Could you check a few things on this drawing? It's one solid part, dimensions in mm from its lowest x, y, z. A direction names the side the tool comes from. Coordinates: 2 decimals unless noted, no trailing zeros. Order: outer loops, then holes, each group sorted by start corner. A loop starts at its lowest first (then second) coordinate and runs counter-clockwise, first axis right, second up. Notation, with made-up numbers: (56.25, 76.25) - (111.25, 76.25) arc R20 cw to (111.25, 112.25) - close; hole circle Ø4 at (8, 64). An arc over 180 degrees is marked (long way). Return JSON: item names as keys, results as strings. Group by question number.
1) Imagine slicing it at A-A (z = 6). Write out the boundary of the cut face in (x, y).
2) Which directions (+Z, -Z, +X, -X, +Y, -Y) give clear straight access to the entire face, cutting with the end or side of a thin tool? Please do the marked faces 1 and 2.
3) Imagine slicing it at B-B (y = 6.25). Write out the boundary of the cut face in (x, z), and give its area (3 significant figures).
4) For pin 1 Ø6 at (y, z) = (2.5, 21.5) entering from +X; pin 2 Ø10 at (x, z) = (8, 23.5) entering from -Y; pin 3 Ø4 at (y, z) = (5.5, 60) entering from +X, each with a flat end and sliding along its axis, tell me the tip position at first contact or that it passes through.
5) If we mould it in two halves opening along Y, with no side actions, what happens to the marked faces 3, 4 and 5? For each: pulls with the +Y half, pulls with the -Y half, needs draft (parallel to the pull), parting line crosses it, or undercut.
6) If I drill on line 1 along Y through (x, z) = (43, 43); line 2 along Y through (x, z) = (16, 51.5); line 3 along X through (y, z) = (4.75, 20.5), over which ranges is the centre line in solid material (lowest first)?
7) Imagine slicing it at D-D (x = 27.94). Write out the boundary of the cut face in (y, z).
8) Imagine slicing it at C-C (x = 38). Write out the boundary of the cut face in (y, z).
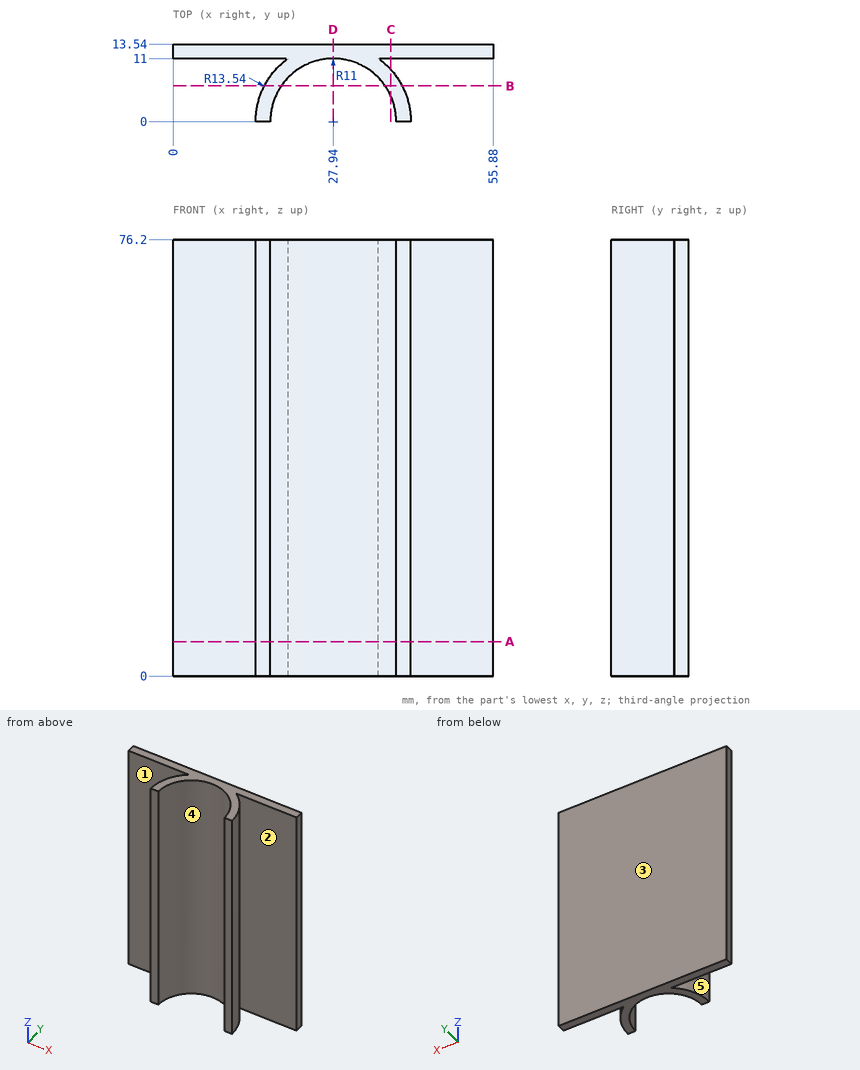
Calculated:
{
 "1": {"outline": "(0, 11) - (20.04, 11) arc R13.54 ccw to (14.4, 0) - (16.94, 0) arc R11 cw to (38.94, 0) - (41.48, 0) arc R13.54 ccw to (35.84, 11) - (55.88, 11) - (55.88, 13.54) - (0, 13.54) - close"},
 "2": {"face 1": "+Z, -Z, -X", "face 2": "+Z, -Z, +X"},
 "3": {"outline": "(15.93, 0) - (18.89, 0) - (18.89, 76.2) - (15.93, 76.2) - close; (36.99, 0) - (39.95, 0) - (39.95, 76.2) - (36.99, 76.2) - close", "area": "451 mm2"},
 "4": {"pin 1": "x = 41.48", "pin 2": "y = 11", "pin 3": "x = 41.02"},
 "5": {"face 3": "pulls with the +Y half", "face 4": "pulls with the -Y half", "face 5": "undercut"},
 "6": {"line 1": "11 to 13.54", "line 2": "0 to 6.38, 11 to 13.54", "line 3": "15.26 to 18.02, 37.86 to 40.62"},
 "7": {"outline": "(11, 0) - (13.54, 0) - (13.54, 76.2) - (11, 76.2) - close"},
 "8": {"outline": "(4.45, 0) - (9.06, 0) - (9.06, 76.2) - (4.45, 76.2) - close; (11, 0) - (13.54, 0) - (13.54, 76.2) - (11, 76.2) - close"}
}
